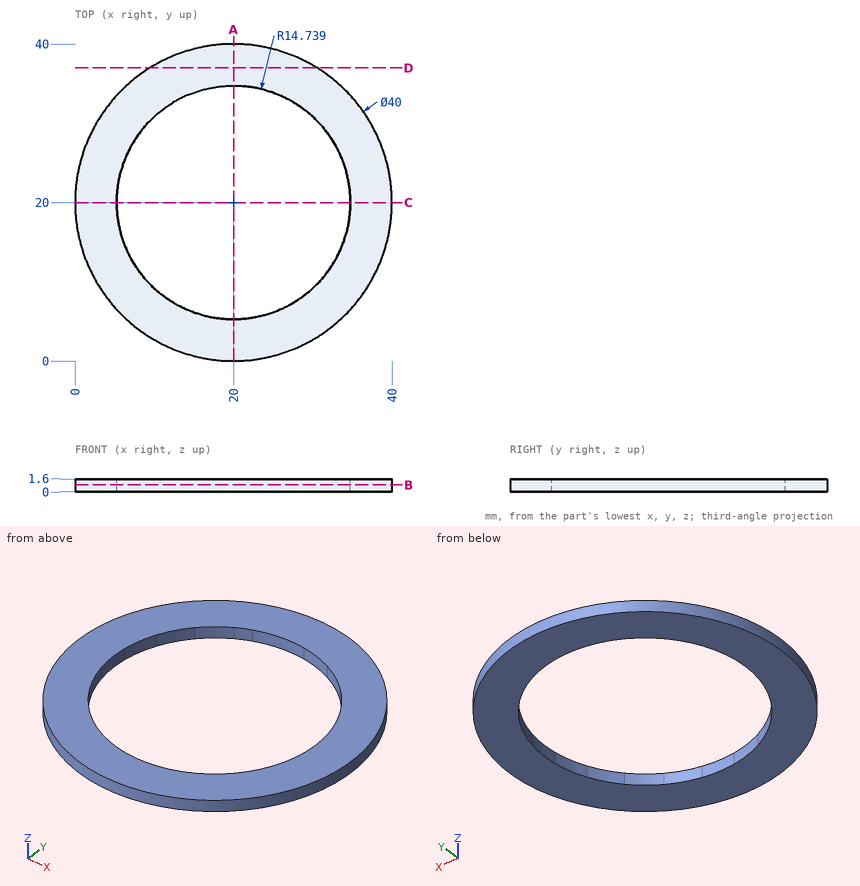
For this review, use the dimensioned drawing (mm, ordinates from the lowest corner) and the shaded views. Give positions to 0.01 mm unless a question says otherwise; leave off trailing zeros. Order: outer loops, then holes, each group sorted by start corner. A loop starts at its lowest first (then second) coordinate and runs counter-clockwise, first axis right, second up. Notation, with made-up numbers: (46, 4.25) - (79, 4.25) arc R16 cw to (79, 31.25) - close; hole circle Ø4 at (89, 49.5). An arc over 180 degrees is marked (long way). Write item = value, one per line. Start each with the question number.
Q1. We need section B-B on z = 0.85. State the section outline as (x, y) points (1 decimal).
Q2. We need section A-A on x = 20. State the section outline as (y, z) points.
Q3. To check wall thickness, follow L1, parallel to X at y = 33.5, z = 1.3 (1 decimal); L2, parallel to Y at x = 27, z = 0.25 (1 decimal); L3, parallel to Y at x = 25, z = 0.5 (1 decimal). State the ranges of each line that lie inside material, in increasing order. Write a range as from..to.
Q4. We need section D-D on y = 37. State the section outline as (x, z) points (1 decimal).
Q5. Clearance check with a flat-ended pin moving along its axis: pin 1 Ø3 at (x, y) = (12, 12) entering from -Z. State where the tip first meets the part, or that it passes through.
Working result:
q1.outline = circle Ø40 at (20, 20); hole circle Ø29.5 at (20, 20)
q2.outline = (0, 0) - (5.26, 0) - (5.26, 1.6) - (0, 1.6) - close; (34.74, 0) - (40, 0) - (40, 1.6) - (34.74, 1.6) - close
q3.L1 = 5.2..14.1, 25.9..34.8
q3.L2 = 1.3..7, 33..38.7
q3.L3 = 0.6..6.1, 33.9..39.4
q4.outline = (9.5, 0) - (30.5, 0) - (30.5, 1.6) - (9.5, 1.6) - close
q5.pin_1 = through
